Geometry check sheet. Reference: the model listing, model coordinates, mm. Face numbers are marked on the shaded views. A direction names the side the tool comes from. Round coordinates to 2 decimals unless told otherwise and drop trailing zeros. Order: outer loops, then holes, each group sorted by start corner. A loop starts at its lowest first (then second) coordinate and runs counter-clockwise, first axis right, second up.
(1) Set-up check for the marked faces 1 and 2: record each of +Z, -Z, +X, -X, +Y, -Y from which the full face is reachable in a straight line by a thin tool's end or side.
(2) Sectioned sample at D-D (z = -63). Record the boundary of the cut face in (x, y), plus the area to 3 significant figures.
(3) Sectioned sample at C-C (y = 6). Record the boundary of the cut face in (x, z).
(4) Go/stop test with flat-tipped pins: pin 1 (2.5 mm diameter, centred on y = 1, z = -33.5, fed in from +X); pin 2 (3.5 mm diameter, centred on y = 1, z = -41.5, fed in from -X); pin 3 (21 mm diameter, centred on x = 35, z = -45.5, fed in from -Y). Record where each tip stops, or that it passes through.
(5) Material ranges on line 1 along X through (y, z) = (1.9, -35); line 2 along X through (y, z) = (6.4, -35); line 3 along Y through (x, z) = (14, -35), recorded low to high.
(6) Sectioned sample at A-A (z = -35). Record the boundary of the cut face in (x, y), plus the area to 3 significant figures.
(7) Sectioned sample at B-B (x = 35). Record the boundary of the cut face in (y, z).
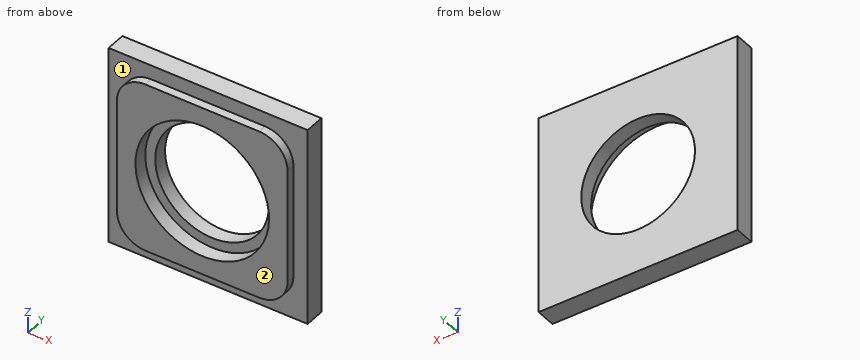
from build123d import *

# Parameters (mm, degrees)
SZKIC1_W                    = 70
SZKIC1_H                    = 70
SZKIC1_R                    = 20
DODANIE_WYCI_GNI_CIE1_DEPTH = 10
SZKIC1_3_W                  = 70
SZKIC1_3_H                  = 70
WYTNIJ_WYCI_GNI_CIE1_DEPTH  = 3
SZKIC1_4_R                  = 23.5
SZKIC1_4_R_2                = 20
WYTNIJ_WYCI_GNI_CIE2_DEPTH  = 5


with BuildPart() as part:
    # Szkic1 → Dodanie-wyci_gni_cie1 (new body)
    with BuildSketch(Plane(origin=(0, 0, 0), x_dir=(1, 0, 0), z_dir=(0, 1, 0))):
        with Locations((35, 35)):
            Rectangle(SZKIC1_W, SZKIC1_H)
        with Locations(Location((35, 35, 0), (0, 0, 270))):
            Circle(SZKIC1_R, mode=Mode.SUBTRACT)
    extrude(amount=DODANIE_WYCI_GNI_CIE1_DEPTH)

    # Szkic1_3 → Wytnij-wyci_gni_cie1 (cut)
    with BuildSketch(Plane(origin=(0, 0, 0), x_dir=(1, 0, 0), z_dir=(0, 1, 0))):
        with Locations((35, 35)):
            Rectangle(SZKIC1_3_W, SZKIC1_3_H)
        with BuildLine():
            Line((5, 35), (5, 55))
            ThreePointArc((5, 55), (7.928932188, 62.071067812), (15, 65))
            Line((15, 65), (55, 65))
            ThreePointArc((55, 65), (62.071067812, 62.071067812), (65, 55))
            Line((65, 55), (65, 15))
            ThreePointArc((65, 15), (62.071067812, 7.928932188), (55, 5))
            Line((55, 5), (15, 5))
            ThreePointArc((15, 5), (7.928932188, 7.928932188), (5, 15))
            Line((5, 15), (5, 35))
        make_face(mode=Mode.SUBTRACT)
    extrude(amount=WYTNIJ_WYCI_GNI_CIE1_DEPTH, mode=Mode.SUBTRACT)

    # Szkic1_4 → Wytnij-wyci_gni_cie2 (cut)
    with BuildSketch(Plane(origin=(0, 0, 0), x_dir=(1, 0, 0), z_dir=(0, 1, 0))):
        with Locations(Location((35, 35, 0), (0, 0, 270))):
            Circle(SZKIC1_4_R)
        with Locations(Location((35, 35, 0), (0, 0, 270))):
            Circle(SZKIC1_4_R_2, mode=Mode.SUBTRACT)
    extrude(amount=WYTNIJ_WYCI_GNI_CIE2_DEPTH, mode=Mode.SUBTRACT)


solid = part.part
Answer below:
1. face 1: -Y
1. face 2: +Z, -Z, +X, -X, -Y
2. outline: (0, 3) - (9, 3) - (9, 0) - (61, 0) - (61, 3) - (70, 3) - (70, 10) - (0, 10) - close
2. area: 646 mm2
3. outline: (0, -70) - (70, -70) - (70, 0) - (0, 0) - close; hole circle Ø40 at (35, -35)
4. pin 1: stops at x = 65
4. pin 2: stops at x = 5
4. pin 3: stops at y = 5
5. line 1: x = 5 to 11.5, 58.5 to 65
5. line 2: x = 0 to 15, 55 to 70
5. line 3: y = 5 to 10
6. outline: (0, 3) - (5, 3) - (5, 0) - (11.5, 0) - (11.5, 5) - (15, 5) - (15, 10) - (0, 10) - close; (55, 5) - (58.5, 5) - (58.5, 0) - (65, 0) - (65, 3) - (70, 3) - (70, 10) - (55, 10) - close
6. area: 235 mm2
7. outline: (0, -65) - (3, -65) - (3, -70) - (10, -70) - (10, -55) - (5, -55) - (5, -58.5) - (0, -58.5) - close; (0, -11.5) - (5, -11.5) - (5, -15) - (10, -15) - (10, 0) - (3, 0) - (3, -5) - (0, -5) - close
